Job drawing, mm, ordinate dimensions from the low corner. One solid piece. A direction names the side the tool comes from. Round coordinates to 2 decimals unless told otherwise and drop trailing zeros. Write each loop counter-clockwise with the first axis right and the second up, starting at its lowest first coordinate (ties: lowest second). Pieces come first, ordered by that corner, then holes. Notation, with made-up numbers: (41.25, 84) -> (58.25, 84) arc R25 ccw to (58.25, 122) -> close; hole circle Ø5 at (12.25, 66). An arc over 180 degrees is marked (long way). Use CSV: the item, a comma, the result in double quotes. Start each with the question number.
(1) Which spindle directions (+Z, -Z, +X, -X, +Y, -Y) get a long thin tool onto all of the face, cutting with end or side? Do the marked faces 1, 2 and 3. Say none if no direction does.
(2) Saw through at C-C (z = 9.5). Give the cut face in (x, y) (1 decimal), plus the area to 3 significant figures.
(3) Saw through at B-B (x = 15). Give the cut face in (y, z).
(4) Saw through at D-D (y = 32). Give the cut face in (x, z).
(5) Probe line 1 (Y direction, x = 37, z = 4) (1 decimal); line 2 (X direction, y = 55, z = 33) (1 decimal); line 3 (Z direction, x = 86, y = 35.5). List the from-to ranges inside material, lowest first. Write a range as [from, to].
(6) Saw through at A-A (y = 10.5). Give the cut face in (x, z).
(7) Two-plate mould, pull along X, no slides. Class the marked faces 4, 5, 6 and 7: released by +X, released by -X, zero draft, split by the parting line, or undercut.
(8) Drop flat-ended pins along their axis: pin 1 (8 mm diameter, centred on y = 50.5, z = 40, fed in from -X); pin 2 (5 mm diameter, centred on x = 14, y = 34.5, fed in from +Z); pin 3 (14 mm diameter, centred on x = 63, z = 42.5, fed in from -Y); pin 4 (2 mm diameter, centred on x = 32.5, y = 30, fed in from +Z). Give the stop position or say it passes through.
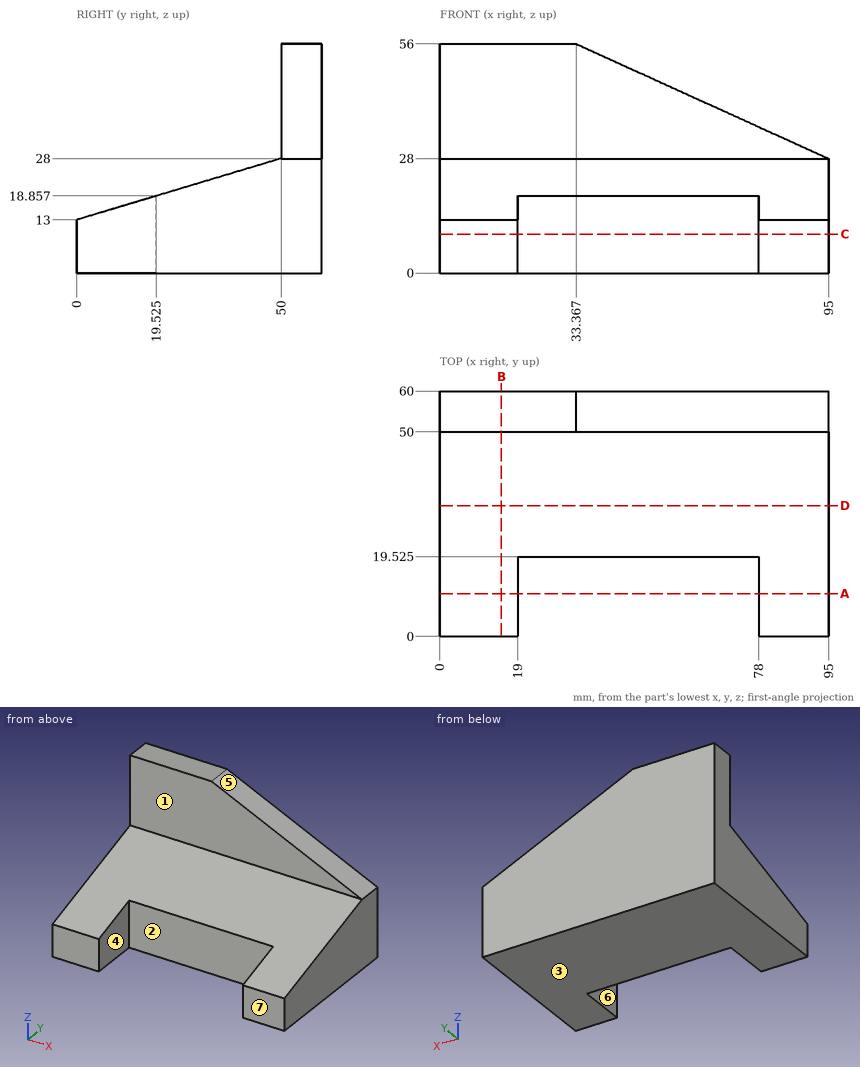
Answers:
1,face 1,"+Z, +X, -X, -Y"
1,face 2,"+Z, -Z, -Y"
1,face 3,"-Z, +X, -X, +Y, -Y"
2,outline,"(0, 0) -> (19, 0) -> (19, 19.5) -> (78, 19.5) -> (78, 0) -> (95, 0) -> (95, 60) -> (0, 60) -> close"
2,area,"4,550 mm²"
3,outline,"(0, 0) -> (60, 0) -> (60, 56) -> (50, 56) -> (50, 28) -> (0, 13) -> close"
4,outline,"(0, 0) -> (95, 0) -> (95, 22.6) -> (0, 22.6) -> close"
5,line 1,"y = [19.5, 60]"
5,line 2,"x = [0, 84]"
5,line 3,"z = [0, 23.65]"
6,outline,"(0, 0) -> (19, 0) -> (19, 16.15) -> (0, 16.15) -> close; (78, 0) -> (95, 0) -> (95, 16.15) -> (78, 16.15) -> close"
7,face 4,"undercut"
7,face 5,"released by +X"
7,face 6,"undercut"
7,face 7,"zero draft"
8,pin 1,"stops at x = 0"
8,pin 2,"stops at z = 24.1"
8,pin 3,"stops at y = 50"
8,pin 4,"stops at z = 22.3"
